The model under review builds one solid part; all positions refer to its coordinate system, in mm. Face numbers are marked on the shaded views. A direction names the side the tool comes from. Give positions to 0.01 mm unless a question says otherwise; leave off trailing zeros. Order: outer loops, then holes, each group sorted by start corner. A loop starts at its lowest first (then second) coordinate and runs counter-clockwise, first axis right, second up. Notation, with made-up numbers: (74, 84) - (106, 84) arc R12 ccw to (106, 90) - close; hole circle Ø2 at (47, 8). An arc over 180 degrees is marked (long way). Answer as CSV lines item,"result". Start each with the question number.
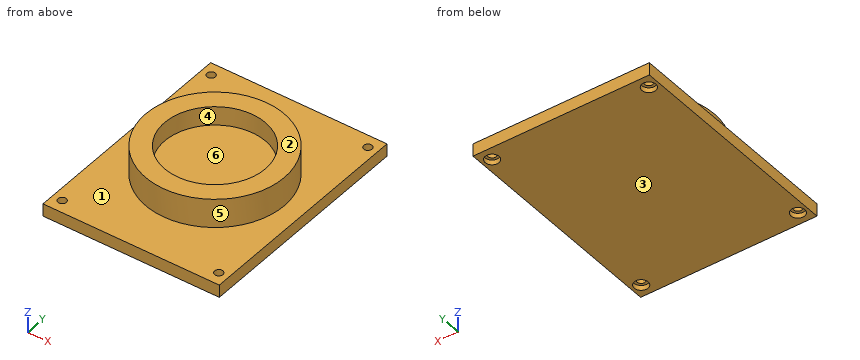
from build123d import *

# Parameters (mm, degrees)
CROQUIS1_W                                           = 140
CROQUIS1_H                                           = 180
SALIENTE_EXTRUIR1_DEPTH                              = 10
CROQUIS2_R                                           = 55
SALIENTE_EXTRUIR2_DEPTH                              = 8
CROQUIS3_R                                           = 55
CROQUIS3_R_2                                         = 40
SALIENTE_EXTRUIR3_DEPTH                              = 15
REFRENTADO_PARA_TORNILLO_CON_CABEZA_PLAN_D           = 6.6
REFRENTADO_PARA_TORNILLO_CON_CABEZA_PLAN_CBORE_D     = 11
REFRENTADO_PARA_TORNILLO_CON_CABEZA_PLAN_CBORE_DEPTH = 3.9


with BuildPart() as part:
    # Croquis1 → Saliente-Extruir1 (new body)
    with BuildSketch(Plane.XY):
        with Locations((70, 90)):
            Rectangle(CROQUIS1_W, CROQUIS1_H)
    extrude(amount=SALIENTE_EXTRUIR1_DEPTH)

    # Croquis2 → Saliente-Extruir2 (add)
    with BuildSketch(Plane.XY.offset(10)):
        with Locations((70, 90)):
            Circle(CROQUIS2_R)
    extrude(amount=SALIENTE_EXTRUIR2_DEPTH)

    # Croquis3 → Saliente-Extruir3 (add)
    with BuildSketch(Plane.XY.offset(18)):
        with Locations((70, 90)):
            Circle(CROQUIS3_R)
        with Locations((70, 90)):
            Circle(CROQUIS3_R_2, mode=Mode.SUBTRACT)
    extrude(amount=SALIENTE_EXTRUIR3_DEPTH)

    # Refrentado para tornillo con cabeza plana de M61 (through all)
    with Locations(Plane(origin=(0, 0, 0), x_dir=(-1, 0, 0), z_dir=(0, 0, -1))):
        with Locations((-132.222222222, 170), (-7.777777778, 170), (-7.777777778, 10), (-132.222222222, 10)):
            CounterBoreHole(REFRENTADO_PARA_TORNILLO_CON_CABEZA_PLAN_D / 2, REFRENTADO_PARA_TORNILLO_CON_CABEZA_PLAN_CBORE_D / 2, REFRENTADO_PARA_TORNILLO_CON_CABEZA_PLAN_CBORE_DEPTH)


solid = part.part
Item 1: Take a section at C-C on y = 90. Write out the cut boundary in (x, z).
Item 2: Mouldability with a two-part tool opening along Y and no side actions: class the marked faces 3, 4, 5 and 6 as released by +Y, released by -Y, zero draft, split by the parting line, or undercut.
Item 3: Take a section at B-B on x = 70. Write out the cut boundary in (y, z).
Item 4: Take a section at D-D on z = 15.5. Write out the cut boundary in (x, y).
Item 5: Machinability: for the marked faces 1 and 2, which of the approach directions +Z, -Z, +X, -X, +Y, -Y give a long, thin tool a straight path to every point of the face, cutting with its end or side? Answer none if there is none.
Item 6: Clearance check with flat-ended pins moving along their axes: pin 1 (8.5 mm diameter, centred on x = 132.22, y = 170, fed in from -Z); pin 2 (5.5 mm diameter, centred on x = 134.5, y = 172.5, fed in from -Z); pin 3 (4 mm diameter, centred on x = 7.78, y = 170, fed in from -Z); pin 4 (1 mm diameter, centred on x = 85, z = 20.5, fed in from -Y). State where each tip first meets the part, or that it passes through.
Item 7: Take a section at A-A on y = 10. Write out the cut boundary in (x, z), and give its area (3 significant figures).
Item 8: For line 1 along Y through (x, z) = (127.5, 3.5); line 2 along Z through (x, y) = (94, 152); line 3 along Z through (x, y) = (99, 87.5), list the stretches that pass through material, from the lowest coordinate up.
Data:
1,outline,"(0, 0) - (140, 0) - (140, 10) - (125, 10) - (125, 33) - (110, 33) - (110, 18) - (30, 18) - (30, 33) - (15, 33) - (15, 10) - (0, 10) - close"
2,face 3,"zero draft"
2,face 4,"undercut"
2,face 5,"split by the parting line"
2,face 6,"undercut"
3,outline,"(0, 0) - (180, 0) - (180, 10) - (145, 10) - (145, 33) - (130, 33) - (130, 18) - (50, 18) - (50, 33) - (35, 33) - (35, 10) - (0, 10) - close"
4,outline,"circle Ø110 at (70, 90)"
5,face 1,"+Z"
5,face 2,"+Z, +X, -X, +Y, -Y"
6,pin 1,"stops at z = 3.9"
6,pin 2,"stops at z = 0"
6,pin 3,"passes through"
6,pin 4,"stops at y = 36.95"
7,outline,"(0, 0) - (2.28, 0) - (2.28, 3.9) - (4.48, 3.9) - (4.48, 10) - (0, 10) - close; (11.08, 3.9) - (13.28, 3.9) - (13.28, 0) - (126.72, 0) - (126.72, 3.9) - (128.92, 3.9) - (128.92, 10) - (11.08, 10) - close; (135.52, 3.9) - (137.72, 3.9) - (137.72, 0) - (140, 0) - (140, 10) - (135.52, 10) - close"
7,area,"1,230 mm^2"
8,line 1,"y = 0 to 7.18, 12.82 to 167.18, 172.82 to 180"
8,line 2,"z = 0 to 10"
8,line 3,"z = 0 to 18"
